Input: part model. Units: mm. Frame: model coordinates. Face numbers are marked on the shaded views. A direction names the side the tool comes from. Coordinates: 2 decimals unless noted, no trailing zeros.
1) Pin query (flat end, axial travel): pin 1 Ø6 at (x, y) = (3, -33.5) entering from -Z; pin 2 Ø2 at (x, y) = (-26, 26.5) entering from -Z; pin 3 Ø10 at (x, y) = (-29.5, -30) entering from +Z. Return the tip coordinate at first contact, or that it passes through.
2) Section query A-A (x = 0). State how many separate pieces and enclosed holes the cut face has, then the cut area to 3 significant figures.
3) Line query: L1, parallel to Z at x = 0, y = 39; L2, parallel to Y at x = -15.5, z = -4.5; L3, parallel to Y at x = 4, z = 101. Output: solid intervals per line, ascending.
4) Draft query along Y for the marked faces 4, 5, 6 and 7. Return one class per face: pulls with the +Y half, pulls with the -Y half, needs draft (parallel to the pull), parting line crosses it, or undercut.
5) Set-up query: the marked faces 1, 2 and 3. Return all of +Z, -Z, +X, -X, +Y, -Y with unobstructed straight access to the full face (end or side cutting, diameter ignored); none if empty.
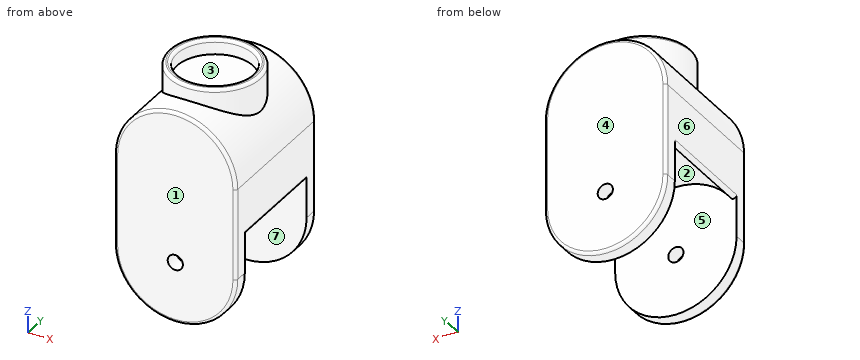
Autodesk Inventor part; units mm, degrees
ref_plane "Work Plane1" through (40, 0, 60) normal (0, 0, -1) x (0, -1, 0)
ref_plane "YZ Plane" through (0, 0, 0) normal (1, 0, 0) x (0, 1, 0)
ref_plane "XZ Plane" through (0, 0, 0) normal (0, 1, 0) x (-1, 0, 0)
sketch "Sketch1" plane through (0, 0, 0) normal (0, 1, 0) x (-1, 0, 0)
  arc A0 (26.4575, 30) -> (-26.4575, 30) centre (0, 0) ccw construction
  arc A1 (40, 60) -> (-40, 60) centre (0, 60) ccw
  line L0 (0, 100) -> (0, 0) construction
  line L1 (40, 60) -> (40, 0)
  line L2 (-40, 60) -> (-40, 0)
  arc A2 (26.4575, 30) -> (40, 60) centre (0, 60) ccw construction
  arc A3 (40, 0) -> (26.4575, 30) centre (0, 0) ccw construction
  arc A4 (-40, 60) -> (26.4575, 30) centre (0, 60) ccw construction
  arc A5 (-26.4575, 30) -> (-40, 0) centre (0, 0) ccw construction
  arc A6 (-40, 0) -> (40, 0) centre (0, 0) ccw
  circle A7 centre (0, 0) radius 5
  dimension "d0" = 80
  dimension "d1" = 80
  dimension "d2" = 100
  dimension "d3" = 10
extrude "Extrusion1" add sketch "Sketch1" along normal mid plane 90
sketch "Sketch2" plane through (0, 0, 0) normal (0, 1, 0) x (-1, 0, 0)
  circle A0 centre (0, 0) radius 5
  circle A1 centre (0, 0) radius 45
  dimension "d6" = 90
extrude "Extrusion2" cut sketch "Sketch2" along normal mid plane 70
fillet "Fillet1" radius 2 10 edges at (40, 0, 20.6155) (-40, 0, 20.6155) (0, 45, -40) (-40, 45, 30) (0, 45, 100) (40, 45, 30) (0, -45, 100) (-40, -45, 30) (0, -45, -40) (40, -45, 30)
ref_plane "Work Plane1" through (40, 0, 60) normal (0, 0, -1) x (0, -1, 0)
sketch "Sketch3" plane through (40, 0, 60) normal (0, 0, -1) x (0, -1, 0)
  circle A0 centre (0, 40) radius 30
  line L0 (0, 40) -> (0, 40)
  dimension "d10" = 60
  dimension "d11" = 0
extrude "Extrusion3" add sketch "Sketch3" against normal blind 50
sketch "Sketch4" plane through (0, 0, 110) normal (0, 0, 1) x (1, 0, 0)
  circle A0 centre (0, 0) radius 30
  circle A1 centre (0, 0) radius 25
  point P0 (0, 0)
  dimension "d14" = 50
extrude "Extrusion4" cut sketch "Sketch4" against normal blind 10 contours A1
fillet "Fillet2" radius 2 2 edges at (0, 30, 110) (-25, 0, 110)
properties part number "Wirst2_V0.4"
Answer:
1. pin 1: stops at z = -40
1. pin 2: stops at z = 36
1. pin 3: stops at z = 91.62
2. separate pieces: 3
2. enclosed holes: 0
2. area: 6,540 mm2
3. L1: z = -40 to -5, 5 to 100
3. L2: y = -45 to -35, 35 to 45
3. L3: y = -29.73 to -24.68, 24.68 to 29.73
4. face 4: pulls with the +Y half
4. face 5: undercut
4. face 6: needs draft
4. face 7: undercut
5. face 1: +Z, -Z, +X, -X, -Y
5. face 2: -Z
5. face 3: +Z
